Can you work these out from the model? Positions are in its coordinate system, mm. Face numbers are marked on the shaded views. A direction names the side the tool comes from. Round coordinates to 2 decimals unless told otherwise and drop trailing zeros. Write each loop counter-clockwise with the first axis right and the second up, starting at its lowest first coordinate (ties: lowest second). Pieces come first, ordered by that corner, then holes. Notation, with made-up numbers: (-22, 84) - (29, 84) arc R19 ccw to (29, 107) - close; hole circle Ø10 at (-6, 54). An arc over 180 degrees is marked (long way). One line per item, written item: value. Start each with the question number.
(1) On a 3-axis mill with a long thin cutter (end or side, diameter ignored), from which of +Z, -Z, +X, -X, +Y, -Y can I reach the whole of each face in a straight line? I mean the marked faces 1 and 2. Say none if no direction works.
(2) I want a section at C-C on y = 6.5. List the corners of the cut face in (x, z) for me (3 decimals).
(3) Thinking about a two-plate mould opening in X: for the marked faces 3, 4 and 5, which applies, +X half, -X half, draft (parallel to the pull), parting line (faces both ways), or undercut?
(4) I'm going to push flat-ended pins straight in: pin 1 Ø4 at (x, z) = (0, 9.525) entering from +Y; pin 2 Ø4 at (x, y) = (1, 7.5) entering from +Z. Where does each tip first touch, or does it pass through?
(5) If I drill on L1, parallel to Z at x = -4.5, y = 5.75 (3 decimals); L2, parallel to Y at x = 0.5, z = 4; L3, parallel to X at y = 1, z = 10.5, over which ranges is the centre line in solid material (lowest first)? Write a range as from..to.
(6) I want a section at B-B on x = -2.75. List the corners of the cut face in (y, z) for me (3 decimals).
(7) I want a section at A-A on x = 0. List the corners of the cut face in (y, z) for me (3 decimals).
(8) I want a section at D-D on z = 3. List the corners of the cut face in (x, y) for me, plus the area to 3 significant figures.
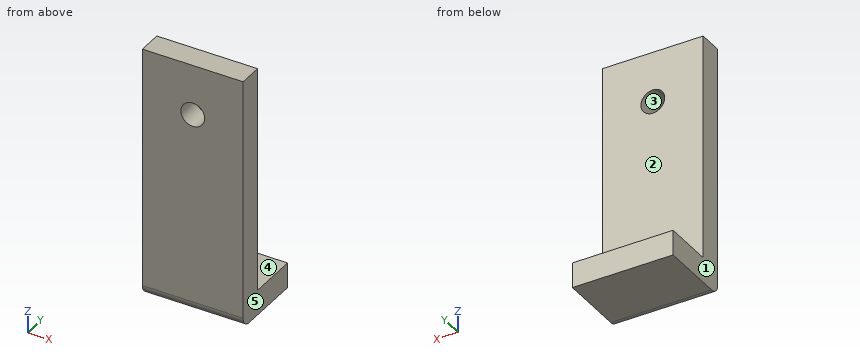
from build123d import *

# Parameters (mm, degrees)
BOSS_EXTRUDE1_DEPTH = 6.35
SKETCH4_R           = 1.5
CUT_EXTRUDE1_DEPTH  = 19.238986403
FILLET1_R           = 1.27


with BuildPart() as part:
    # Sketch1 → Boss-Extrude1 (new, symmetric)
    with BuildSketch(Plane(origin=(0, 0, 0), x_dir=(0, 0, -1), z_dir=(1, 0, 0))):
        Polygon((-15.875, 0), (15.875, 0), (15.875, 9.398), (12.7, 9.398), (12.7, 3.048), (-15.875, 3.048), align=None)
    extrude(amount=BOSS_EXTRUDE1_DEPTH, both=True)

    # Sketch4 → Cut-Extrude1 (cut, through all)
    with BuildSketch(Plane(origin=(0, 3.048, 0), x_dir=(1, 0, 0), z_dir=(0, 1, 0))):
        with Locations(Location((0, -9.525, 0), (0, 0, 270))):
            Circle(SKETCH4_R)
    extrude(amount=-CUT_EXTRUDE1_DEPTH, mode=Mode.SUBTRACT)

    # Fillet1
    fillet1_edges = [part.edges().sort_by_distance(p)[0] for p in [
        (0, 0, -15.875),
    ]]
    fillet(fillet1_edges, radius=FILLET1_R)


solid = part.part
Established:
1. face 1: +Z, -Z, -X, +Y, -Y
1. face 2: +Z, +X, -X, +Y
2. outline: (-6.35, -15.875) - (6.35, -15.875) - (6.35, -12.7) - (-6.35, -12.7) - close
3. face 3: undercut
3. face 4: draft
3. face 5: +X half
4. pin 1: y = 3.05
4. pin 2: z = -12.7
5. L1: -15.875..-12.7
5. L2: 0..3.05
5. L3: -6.35..-1.14, 1.14..6.35
6. outline: (0, -14.605) arc R1.27 ccw to (1.27, -15.875) - (9.398, -15.875) - (9.398, -12.7) - (3.048, -12.7) - (3.048, 15.875) - (0, 15.875) - close
7. outline: (0, -14.605) arc R1.27 ccw to (1.27, -15.875) - (9.398, -15.875) - (9.398, -12.7) - (3.048, -12.7) - (3.048, 8.025) - (0, 8.025) - close; (0, 11.025) - (3.048, 11.025) - (3.048, 15.875) - (0, 15.875) - close
8. outline: (-6.35, 0) - (6.35, 0) - (6.35, 3.05) - (-6.35, 3.05) - close
8. area: 38.7 mm2
